Here's the drawing with two shaded views (mm, measured from the low corner). I have some questions. A direction names the side the tool comes from. Round coordinates to 2 decimals unless told otherwise and drop trailing zeros. Order: outer loops, then holes, each group sorted by start corner. A loop starts at its lowest first (then second) coordinate and runs counter-clockwise, first axis right, second up.
Q1. If we section it at D-D (z = 14.75): Please give me the cut outline in (x, y).
Q2. Will these pins go through, and if not, where does the flat tip stop? P1, Ø3, axis at x = 9, y = 44, coming from the +Z side; P2, Ø0.5, axis at x = 20, y = 66, coming from the +Z side; P3, Ø3, axis at x = 10.45, y = 66.655, coming from the +Z side; P4, Ø1.1, axis at x = 20.5, y = 37, coming from the +Z side.
Q3. If we section it at B-B (z = 10): Please give me the cut outline in (x, y), plus the area to 3 significant figures.
Q4. We'd pull the mould along X, two halves only. Please class the marked faces 1, 2 and 3: pulls with the +X half, pulls with the -X half, needs draft (parallel to the pull), parting line crosses it, or undercut.
Q5. If I drill on line 1 (Y direction, x = 10.45, z = 2.4) (3 decimals); line 2 (X direction, y = 15, z = 13.75); line 3 (Y direction, x = 6.25, z = 19), over which ranges is the centre line in solid material (lowest first)?
Q6. If we section it at A-A (x = 10.45): Please give me the cut outline in (y, z) (3 decimals), plus the area to 3 significant figures.
Q7. For the marked faces 4 and 5, which set-ups out of +Z, -Z, +X, -X, +Y, -Y let a thin tool reach every point of the face, with its end or its side?
Q8. If we section it at C-C (y = 72): Please give me the cut outline in (x, z).
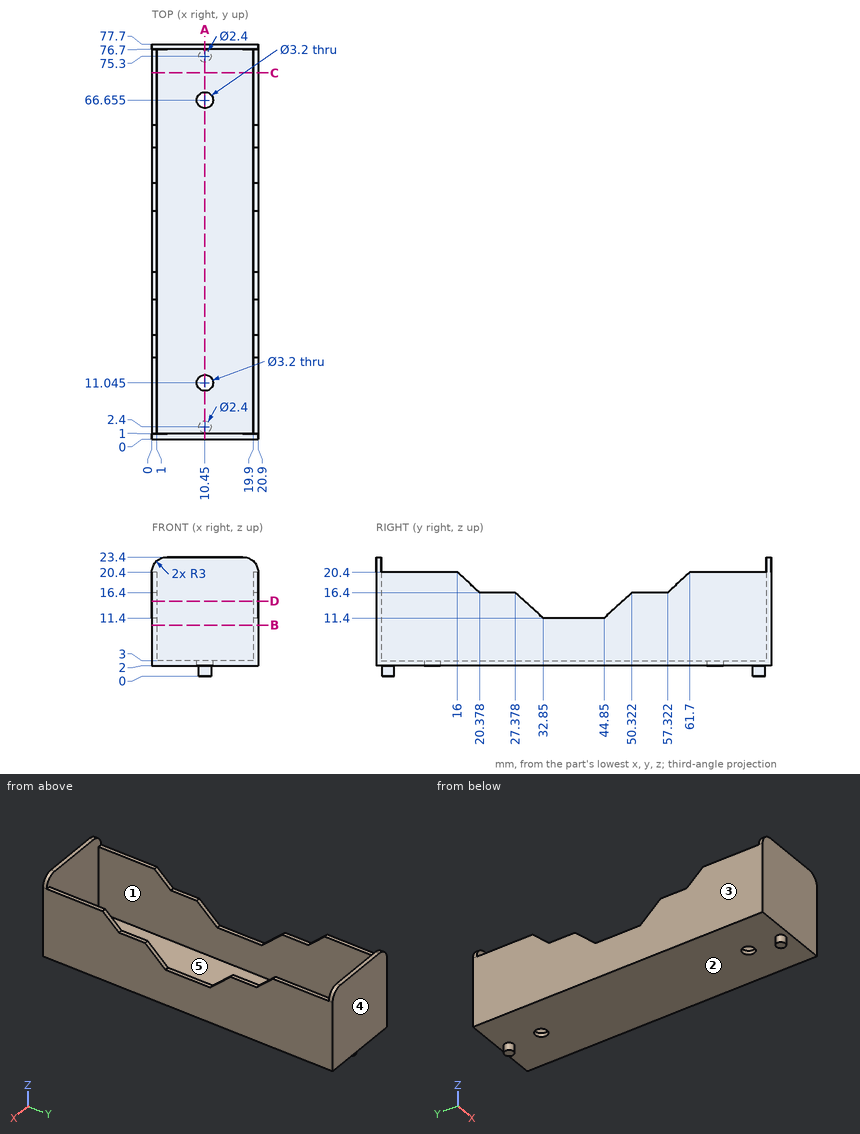
Solution:
1. outline: (0, 0) - (20.9, 0) - (20.9, 29.18) - (19.9, 29.18) - (19.9, 1) - (1, 1) - (1, 29.18) - (0, 29.18) - close; (0, 48.52) - (1, 48.52) - (1, 76.7) - (19.9, 76.7) - (19.9, 48.52) - (20.9, 48.52) - (20.9, 77.7) - (0, 77.7) - close
2. P1: stops at z = 3
2. P2: stops at z = 20.4
2. P3: passes through
2. P4: stops at z = 11.4
3. outline: (0, 0) - (20.9, 0) - (20.9, 77.7) - (0, 77.7) - close; hole (1, 1) - (19.9, 1) - (19.9, 76.7) - (1, 76.7) - close
3. area: 193 mm2
4. face 1: undercut
4. face 2: needs draft
4. face 3: pulls with the -X half
5. line 1: y = 0 to 9.445, 12.645 to 65.055, 68.255 to 77.7
5. line 2: x = 0 to 1, 19.9 to 20.9
5. line 3: y = 0 to 1, 76.7 to 77.7
6. outline: (0, 2) - (1.2, 2) - (1.2, 0) - (3.6, 0) - (3.6, 2) - (9.445, 2) - (9.445, 3) - (1, 3) - (1, 23.4) - (0, 23.4) - close; (12.645, 2) - (65.055, 2) - (65.055, 3) - (12.645, 3) - close; (68.255, 2) - (74.1, 2) - (74.1, 0) - (76.5, 0) - (76.5, 2) - (77.7, 2) - (77.7, 23.4) - (76.7, 23.4) - (76.7, 3) - (68.255, 3) - close
6. area: 122 mm2
7. face 4: +Z, -Z, +X, -X, +Y
7. face 5: +Z
8. outline: (0, 2) - (20.9, 2) - (20.9, 20.4) - (19.9, 20.4) - (19.9, 3) - (1, 3) - (1, 20.4) - (0, 20.4) - close
